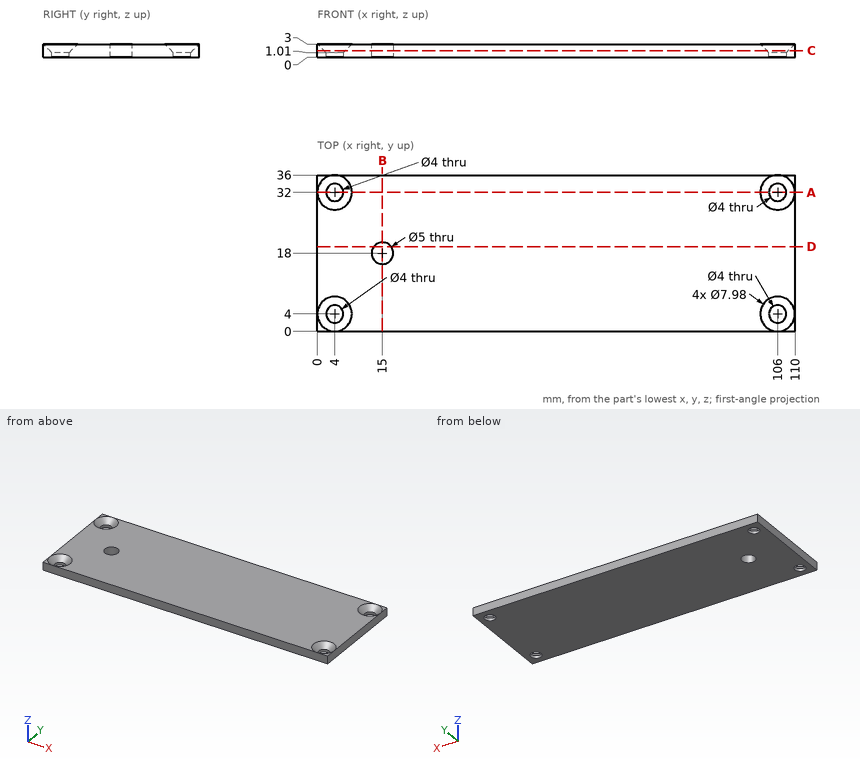
Can you work these out from the drawing? Everything is in mm from the part's minimum corner. Give positions to 0.01 mm unless a question says otherwise; leave off trailing zeros. Loops run counter-clockwise (first coordinate to the right, second up) from the corner with the lowest first, then second, coordinate; pieces in that order, holes last. Notation, with made-up numbers: (82.25, 75) -> (95.25, 75) arc R14 cw to (95.25, 80) -> close; hole circle Ø10 at (-23, 30.25). An arc over 180 degrees is marked (long way). Return JSON: item names as keys, results as strings.
Item 1: I'm going to push a flat-ended pin straight in: pin 1 (6.5 mm diameter, centred on x = 4, y = 4, fed in from +Z). Where does the tip first touch, or does it pass through?
Geometry results:
{"pin 1": "stops at z = 2.26"}
Item 2: If we section it at C-C on z = 1.5: List the corners of the cut face in (x, y) for me, plus the area to 3 significant figures.
Geometry results:
{"outline": "(0, 0) -> (110, 0) -> (110, 36) -> (0, 36) -> close; hole circle Ø4.98 at (4, 4); hole circle Ø4.98 at (4, 32); hole circle Ø5 at (15, 18); hole circle Ø4.98 at (106, 4); hole circle Ø4.98 at (106, 32)", "area": "3,860 mm²"}
Item 3: If we section it at A-A on y = 32: Count the separate pieces of the cut face and the enclosed holes in it, plus the area to 3 significant figures.
Geometry results:
{"separate pieces": "3", "enclosed holes": "0", "area": "298 mm²"}
Item 4: If we section it at D-D on y = 19.5: List the corners of the cut face in (x, z) for me.
Geometry results:
{"outline": "(0, 0) -> (13, 0) -> (13, 3) -> (0, 3) -> close; (17, 0) -> (110, 0) -> (110, 3) -> (17, 3) -> close"}
Item 5: I need wall thicknesses on L1, parallel to Y at x = 106, z = 0.4; L2, parallel to Y at x = 15, z = 2.15; L3, parallel to Y at x = 14.5, z = 2.1. Which ranges of each line are inside material? Lowest first, please. Write a range as from..to.
Geometry results:
{"L1": "y = 0..2, 6..30, 34..36", "L2": "y = 0..15.5, 20.5..36", "L3": "y = 0..15.55, 20.45..36"}
Item 6: If we section it at B-B on x = 15: List the corners of the cut face in (y, z) for me, plus the area to 3 significant figures.
Geometry results:
{"outline": "(0, 0) -> (15.5, 0) -> (15.5, 3) -> (0, 3) -> close; (20.5, 0) -> (36, 0) -> (36, 3) -> (20.5, 3) -> close", "area": "93.0 mm²"}
